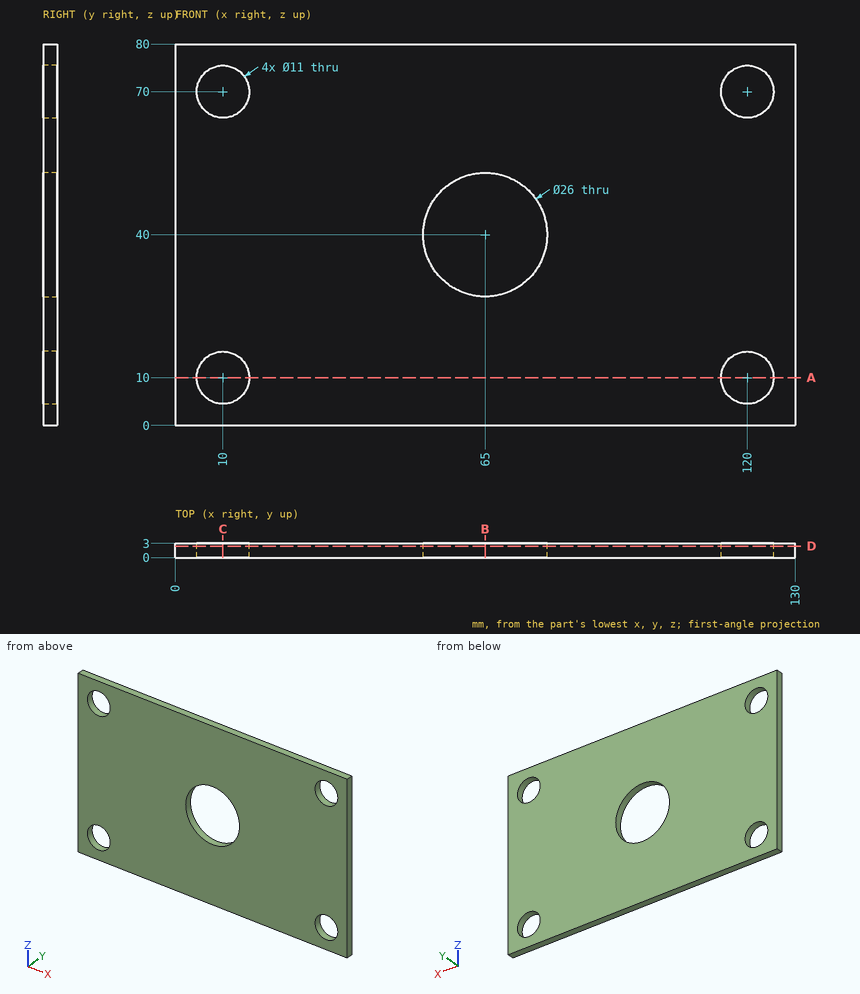
Study the drawing (mm; zero at the part's minimum x, y, z) and answer. Coordinates: 2 decimals unless noted, no trailing zeros. Order: outer loops, then holes, each group sorted by start corner. A loop starts at its lowest first (then second) coordinate and runs counter-clockwise, first axis right, second up. Notation, with made-up numbers: M -31,10 L -14,10 A18 cw -14,37 Z; hole C -14.5,-27 d11. An arc over 180 degrees is marked long. Answer as a JSON object with one key per item and string values. Group by question number.
1. Section A-A on z = 10 is taken. Write down the section's boundary in (x, y).
2. Section D-D on y = 2.4 is taken. Write down the section's boundary in (x, z).
3. A flat-ended cylindrical pin translates along its axis: P1, Ø4, axis at x = 51, z = 47, coming from the -Y side. Find the tip coordinate at first contact, or state that the pin passes through.
4. Straight lines are drawn through the part: line 1 (X direction, y = 1.95, z = 10); line 2 (X direction, y = 0.4, z = 71); line 3 (Z direction, x = 118, y = 1.25). For each, find the intervals that lie inside material, in ascending order.
5. Section C-C on x = 10 is taken. Write down the section's boundary in (y, z).
6. Section B-B on x = 65 is taken. Write down the section's boundary in (y, z), then the cut area to 3 significant figures.
Values follow:
{
 "1": {"outline": "M 0,0 L 4.5,0 L 4.5,3 L 0,3 Z; M 15.5,0 L 114.5,0 L 114.5,3 L 15.5,3 Z; M 125.5,0 L 130,0 L 130,3 L 125.5,3 Z"},
 "2": {"outline": "M 0,0 L 130,0 L 130,80 L 0,80 Z; hole C 10,10 d11; hole C 10,70 d11; hole C 65,40 d26; hole C 120,10 d11; hole C 120,70 d11"},
 "3": {"P1": "y = 0"},
 "4": {"line 1": "0 to 4.5, 15.5 to 114.5, 125.5 to 130", "line 2": "0 to 4.59, 15.41 to 114.59, 125.41 to 130", "line 3": "0 to 4.88, 15.12 to 64.88, 75.12 to 80"},
 "5": {"outline": "M 0,0 L 3,0 L 3,4.5 L 0,4.5 Z; M 0,15.5 L 3,15.5 L 3,64.5 L 0,64.5 Z; M 0,75.5 L 3,75.5 L 3,80 L 0,80 Z"},
 "6": {"outline": "M 0,0 L 3,0 L 3,27 L 0,27 Z; M 0,53 L 3,53 L 3,80 L 0,80 Z", "area": "162 mm2"}
}
